Autodesk Inventor part; units mm, degrees
ref_plane "YZ Plane" through (0, 0, 0) normal (1, 0, 0) x (0, 1, 0)
ref_plane "XZ Plane" through (0, 0, 0) normal (0, 1, 0) x (-1, 0, 0)
ref_plane "XY Plane" through (0, 0, 0) normal (0, 0, 1) x (1, 0, 0)
sketch "Sketch1" plane through (0, 0, 0) normal (0, 1, 0) x (-1, 0, 0)
  line L0 (2, 0) -> (50, 0)
  line L1 (52, -2) -> (52, -146)
  line L2 (50, -148) -> (2, -148)
  line L3 (0, -146) -> (0, -2)
  arc A0 (52, -2) -> (50, 0) centre (50, -2) ccw
  arc A1 (0, -146) -> (2, -148) centre (2, -146) ccw
  arc A2 (50, -148) -> (52, -146) centre (50, -146) ccw
  arc A3 (2, 0) -> (0, -2) centre (2, -2) ccw
  line L4 (52.5, 2.5) -> (-0.5, 2.5)
  line L5 (-2.5, 0.5) -> (-2.5, -148.5)
  line L6 (-0.5, -150.5) -> (52.5, -150.5)
  line L7 (54.5, -148.5) -> (54.5, 0.5)
  arc A4 (54.5, 0.5) -> (52.5, 2.5) centre (52.5, 0.5) ccw
  arc A5 (-0.5, 2.5) -> (-2.5, 0.5) centre (-0.5, 0.5) ccw
  arc A6 (-2.5, -148.5) -> (-0.5, -150.5) centre (-0.5, -148.5) ccw
  arc A7 (52.5, -150.5) -> (54.5, -148.5) centre (52.5, -148.5) ccw
  point P0 (0, 0)
  point P1 (52, -148)
  point P2 (52, 0)
  point P3 (0, -148)
  dimension "d0" = 52
  dimension "d1" = 148
  dimension "d2" = 2
  dimension "d3" = 2.5
  dimension "d4" = 2.5
  dimension "d5" = 2.5
  dimension "d6" = 2.5
  dimension "d7" = 2
extrude "Extrusion1" add sketch "Sketch1" along normal blind 5
sketch "Sketch2" plane through (0, 0, 0) normal (0, -1, 0) x (1, 0, 0)
  arc A0 (2.5, 0.5) -> (0.5, 2.5) centre (0.5, 0.5) ccw
  line L0 (-52.5, 2.5) -> (0.5, 2.5)
  arc A1 (-52.5, 2.5) -> (-54.5, 0.5) centre (-52.5, 0.5) ccw
  line L1 (-54.5, -148.5) -> (-54.5, 0.5)
  arc A2 (-54.5, -148.5) -> (-52.5, -150.5) centre (-52.5, -148.5) ccw
  line L2 (0.5, -150.5) -> (-52.5, -150.5)
  arc A3 (0.5, -150.5) -> (2.5, -148.5) centre (0.5, -148.5) ccw
  line L3 (2.5, 0.5) -> (2.5, -148.5)
  line L4 (0, -146) -> (0, -2)
  arc A4 (-2, -148) -> (0, -146) centre (-2, -146) ccw
  line L5 (-50, -148) -> (-2, -148)
  arc A5 (-52, -146) -> (-50, -148) centre (-50, -146) ccw
  line L6 (-52, -2) -> (-52, -146)
  arc A6 (-50, 0) -> (-52, -2) centre (-50, -2) ccw
  line L7 (-2, 0) -> (-50, 0)
  arc A7 (0, -2) -> (-2, 0) centre (-2, -2) ccw
  line L8 (-49, -146) -> (-3, -146)
  line L9 (-2, -145) -> (-2, -3)
  line L10 (-3, -2) -> (-49, -2)
  line L11 (-50, -3) -> (-50, -145)
  arc A8 (-3, -146) -> (-2, -145) centre (-3, -145) ccw
  arc A9 (-50, -145) -> (-49, -146) centre (-49, -145) ccw
  arc A10 (-49, -2) -> (-50, -3) centre (-49, -3) ccw
  arc A11 (-2, -3) -> (-3, -2) centre (-3, -3) ccw
  point P0 (0, 0)
  dimension "d10" = 1
extrude "Extrusion2" add sketch "Sketch2" along normal blind 2 contours L3 A3 L2 A2 L1 A1 L0 A0 | A4 L5 A5 L6 A6 L7 A7 L4
sketch "Sketch3" plane through (0, -2, 0) normal (0, -1, 0) x (1, 0, 0)
  line L0 (2.5, -148.5) -> (2.5, 0.5)
  arc A0 (2.5, 0.5) -> (0.5, 2.5) centre (0.5, 0.5) ccw
  line L1 (0.5, 2.5) -> (-52.5, 2.5)
  arc A1 (-52.5, 2.5) -> (-54.5, 0.5) centre (-52.5, 0.5) ccw
  line L2 (-54.5, 0.5) -> (-54.5, -148.5)
  arc A2 (-54.5, -148.5) -> (-52.5, -150.5) centre (-52.5, -148.5) ccw
  line L3 (-52.5, -150.5) -> (0.5, -150.5)
  arc A3 (0.5, -150.5) -> (2.5, -148.5) centre (0.5, -148.5) ccw
  arc A4 (-50, -145) -> (-49, -146) centre (-49, -145) ccw
  line L4 (-50, -145) -> (-50, -3)
  arc A5 (-49, -2) -> (-50, -3) centre (-49, -3) ccw
  line L5 (-49, -2) -> (-3, -2)
  arc A6 (-2, -3) -> (-3, -2) centre (-3, -3) ccw
  line L6 (-2, -3) -> (-2, -145)
  arc A7 (-3, -146) -> (-2, -145) centre (-3, -145) ccw
  line L7 (-3, -146) -> (-49, -146)
  point P0 (0, 0)
extrude "Extrusion3" add sketch "Sketch3" along normal blind 2
sketch "Sketch4" plane through (0.5, 5, -150.5) normal (0, 0, -1) x (-1, 0, 0)
  line L0 (-2, -9) -> (-2, 0)
  line L1 (-2, -9) -> (53.9521, -19.876)
  line L2 (-2, -9) -> (54.9993, -9) construction
  line L3 (55, -9) -> (55, 0)
  line L4 (53.9521, -19.876) -> (55, -9)
  line L5 (55, 0) -> (53, 0)
  line L6 (55, 0) -> (53.1086, -19.712)
  point P0 (0.5, -5)
  dimension "d15" = 11
  dimension "d16" = 9
properties part number "hole size and stack size"
Can you work these out from the model? Positions are in its coordinate system, mm. A direction names the side the tool comes from. Give positions to 0.01 mm unless a question says otherwise; leave off trailing zeros. Loops run counter-clockwise (first coordinate to the right, second up) from the corner with the lowest first, then second, coordinate; pieces in that order, holes last. Notation, with made-up numbers: (18, 13.5) -> (25, 13.5) arc R18 cw to (25, 26.5) -> close; hole circle Ø10 at (55, -20.5). An arc over 180 degrees is marked (long way). Return JSON: item names as keys, results as strings.
Q1. I want a section at B-B, the plane z = -117.5. List the corners of the cut face in (x, y) for me, then the cut area to 3 significant figures.
Checks:
{"outline": "(-54.5, -4) -> (-50, -4) -> (-50, 0) -> (-52, 0) -> (-52, 5) -> (-54.5, 5) -> close; (-2, -4) -> (2.5, -4) -> (2.5, 5) -> (0, 5) -> (0, 0) -> (-2, 0) -> close", "area": "61.0 mm2"}
Q2. On a 3-axis mill with a long thin cutter (end or side, diameter ignored), from which of +Z, -Z, +X, -X, +Y, -Y can I reach the whole of each face in a straight line? I mean faces 1 (the face through (-26, 2, 0)), 2 (the face through (-2, -2, -73)), 3 (the face through (-26, 1, 2.5)). Say none if no direction works.
Checks:
{"face 1": "+Y", "face 2": "+Y, -Y", "face 3": "+Z, +X, -X, +Y, -Y"}
Q3. We'd pull the mould along X, two halves only. Please class faces 4 (the face through (-26, -2, -146)), 5 (the face through (-50, -2, -75)), 6 (the face through (-51, -4, -68)), 7 (the face through (2.5, 1, -75)): released by +X, released by -X, zero draft, split by the parting line, or undercut.
Checks:
{"face 4": "undercut", "face 5": "undercut", "face 6": "zero draft", "face 7": "released by +X"}
Q4. I need wall thicknesses on probe 1 along X at (y, z) = (-2.25, -6); probe 2 along Z at (x, y) = (-37, 3.25); probe 3 along X at (y, z) = (2.5, -49). Which ranges of each line are inside material? Lowest first, please.
Checks:
{"probe 1": "x = -54.5 to -50, -2 to 2.5", "probe 2": "z = -150.5 to -148, 0 to 2.5", "probe 3": "x = -54.5 to -52, 0 to 2.5"}
Q5. I want a section at A-A, the plane x = -47. List the corners of the cut face in (y, z) for me, then the cut area to 3 significant figures.
Checks:
{"outline": "(-4, -150.5) -> (5, -150.5) -> (5, -148) -> (0, -148) -> (0, -146) -> (-4, -146) -> close; (-4, -2) -> (0, -2) -> (0, 0) -> (5, 0) -> (5, 2.5) -> (-4, 2.5) -> close", "area": "61.0 mm2"}
